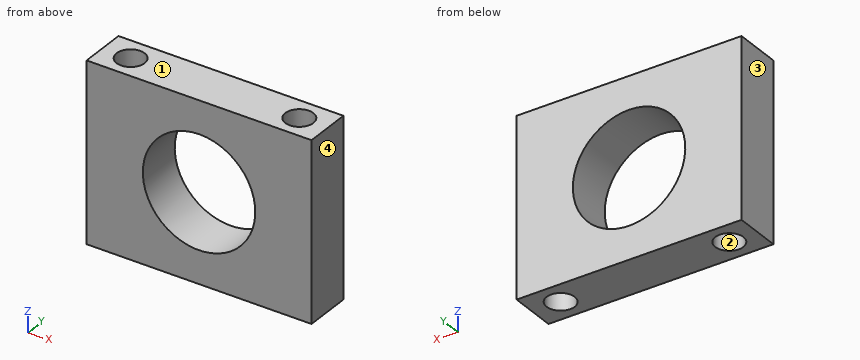
```python
from build123d import *

# Parameters (mm, degrees)
SKETCH_1_W          = 24
SKETCH_1_H          = 19
EXTRUDE_1_DEPTH     = 5
CUT_EXTRUDE_1_REACH = 18.101
SKETCH_2_R          = 6
CUT_EXTRUDE_2_REACH = 25.022
SKETCH_3_R          = 1.5


with BuildPart() as part:
    # 草图1 → 凸台-拉伸1 (new body)
    with BuildSketch(Plane(origin=(0, 0, 0), x_dir=(1, 0, 0), z_dir=(0, 1, 0))):
        Rectangle(SKETCH_1_W, SKETCH_1_H)
    extrude(amount=EXTRUDE_1_DEPTH)

    # 草图2 → 切除-拉伸1 (cut, up to next)
    with BuildSketch(Plane(origin=(0, 5, 0), x_dir=(1, 0, 0), z_dir=(0, 1, 0)), mode=Mode.PRIVATE) as cut_extrude_1_sk1:
        with Locations(Location((0, 0, 0), (0, 0, 270))):
            Circle(SKETCH_2_R)
    cut_extrude_1_tool1 = extrude(cut_extrude_1_sk1.sketch, amount=-CUT_EXTRUDE_1_REACH, mode=Mode.PRIVATE) & part.part
    add(cut_extrude_1_tool1.solids().sort_by_distance((0, 5, 0))[0], mode=Mode.SUBTRACT)

    # 草图3 → 切除-拉伸2 (cut, up to next)
    with BuildSketch(Plane.XY.offset(9.5), mode=Mode.PRIVATE) as cut_extrude_2_sk1:
        with Locations((-9, 2.5)):
            Circle(SKETCH_3_R)
    cut_extrude_2_tool1 = extrude(cut_extrude_2_sk1.sketch, amount=-CUT_EXTRUDE_2_REACH, mode=Mode.PRIVATE) & part.part
    # 草图3 → 切除-拉伸2 (cut, up to next)
    with BuildSketch(Plane.XY.offset(9.5), mode=Mode.PRIVATE) as cut_extrude_2_sk2:
        with Locations((9, 2.5)):
            Circle(SKETCH_3_R)
    cut_extrude_2_tool2 = extrude(cut_extrude_2_sk2.sketch, amount=-CUT_EXTRUDE_2_REACH, mode=Mode.PRIVATE) & part.part
    add(cut_extrude_2_tool1.solids().sort_by_distance((-9, 2.5, 9.5))[0], mode=Mode.SUBTRACT)
    add(cut_extrude_2_tool2.solids().sort_by_distance((9, 2.5, 9.5))[0], mode=Mode.SUBTRACT)


solid = part.part
```
CAD build for the part. Positions are in the model's coordinates, mm. Face numbers are marked on the shaded views. Give positions to 0.01 mm unless a question says otherwise; leave off trailing zeros. Loops run counter-clockwise (first coordinate to the right, second up) from the corner with the lowest first, then second, coordinate; pieces in that order, holes last. Notation, with made-up numbers: (62.25, 44.5) -> (88.25, 44.5) arc R34 cw to (88.25, 79.5) -> close; hole circle Ø6 at (89, -25). An arc over 180 degrees is marked (long way). Use a Markdown table: item, result.
1. Slice it at C-C (y = 2.5). List the corners of the cut face in (x, z).
Check result:
| item | result |
|---|---|
| outline | (-12, -9.5) -> (-10.5, -9.5) -> (-10.5, 9.5) -> (-12, 9.5) -> close; (-7.5, -9.5) -> (7.5, -9.5) -> (7.5, 9.5) -> (-7.5, 9.5) -> close; (10.5, -9.5) -> (12, -9.5) -> (12, 9.5) -> (10.5, 9.5) -> close; hole circle Ø12 at (0, 0) |
2. Slice it at B-B (x = 0). List the corners of the cut face in (y, z).
Check result:
| item | result |
|---|---|
| outline | (0, -9.5) -> (5, -9.5) -> (5, -6) -> (0, -6) -> close; (0, 6) -> (5, 6) -> (5, 9.5) -> (0, 9.5) -> close |
3. Mould opens along X. For the marked faces 1, 2, 3 and 4 say: pulls with the +X half, pulls with the -X half, needs draft (parallel to the pull), parting line crosses it, or undercut.
Check result:
| item | result |
|---|---|
| face 1 | needs draft |
| face 2 | undercut |
| face 3 | pulls with the -X half |
| face 4 | pulls with the +X half |
4. Wall check: L1, parallel to X at y = 2.4, z = -6.75; L2, parallel to X at y = 1.8, z = -1; L3, parallel to Y at x = 9, z = -8.5. Give the ranges that are in metal, low to high. Write a range as [from, to].
Check result:
| item | result |
|---|---|
| L1 | x = [-12, -10.5], [-7.5, 7.5], [10.5, 12] |
| L2 | x = [-12, -10.33], [-7.67, -5.92], [5.92, 7.67], [10.33, 12] |
| L3 | y = [0, 1], [4, 5] |
5. Slice it at A-A (z = 0). List the corners of the cut face in (x, y), plus the area to 3 significant figures.
Check result:
| item | result |
|---|---|
| outline | (-12, 0) -> (-6, 0) -> (-6, 5) -> (-12, 5) -> close; (6, 0) -> (12, 0) -> (12, 5) -> (6, 5) -> close; hole circle Ø3 at (-9, 2.5); hole circle Ø3 at (9, 2.5) |
| area | 45.9 mm^2 |
6. Slice it at D-D (y = 0.7). List the corners of the cut face in (x, z), plus the area to 3 significant figures.
Check result:
| item | result |
|---|---|
| outline | (-12, -9.5) -> (12, -9.5) -> (12, 9.5) -> (-12, 9.5) -> close; hole circle Ø12 at (0, 0) |
| area | 343 mm^2 |
